Could you check a few things on this model? Use its own coordinates, in mm. Give positions to 0.01 mm unless a question says otherwise; leave off trailing zeros. Order: outer loops, then holes, each group sorted by start corner. A loop starts at its lowest first (then second) coordinate and runs counter-clockwise, first axis right, second up. Notation, with made-up numbers: M 48.25,31.25 L 107.25,31.25 A22 ccw 107.25,43.25 Z; hole C 49,85.5 d5. An arc over 180 degrees is marked long. Use a Markdown table: item, result. Add a question column.
Autodesk Inventor part; units mm, degrees
ref_plane "NUT_XY" through (0, 0, 0) normal (0, 0, 1) x (1, 0, 0)
ref_plane "NUT_YZ" through (0, 0, 0) normal (1, 0, 0) x (0, 1, 0)
ref_plane "NUT_ZX" through (0, 0, 0) normal (0, 1, 0) x (0, 0, 1)
sketch "Sketch_8" plane through (0, 0, 0) normal (1, 0, 0) x (0, 1, 0)
  line L0 (0, -4.064) -> (0, 0)
  line L1 (0, 0) -> (5.588, 0)
  line L2 (5.588, 0) -> (6.7056, -0.2995)
  line L3 (6.7056, -0.2995) -> (6.7056, -3.7645)
  line L4 (6.7056, -3.7645) -> (5.588, -4.064)
  line L5 (5.588, -4.064) -> (0, -4.064)
  line L6 (0, -4.064) -> (0, 0)
sketch "Sketch_10" plane through (0, 0, 0) normal (0, 0, 1) x (1, 0, 0)
  line L0 (-11.176, 11.176) -> (-11.176, -11.176)
  line L1 (-11.176, -11.176) -> (11.176, -11.176)
  line L2 (11.176, -11.176) -> (11.176, 11.176)
  line L3 (11.176, 11.176) -> (-11.176, 11.176)
  line L4 (-5.588, 3.2262) -> (-5.588, -3.2262)
  line L5 (-5.588, -3.2262) -> (0, -6.4525)
  line L6 (0, -6.4525) -> (5.588, -3.2262)
  line L7 (5.588, -3.2262) -> (5.588, 3.2262)
  line L8 (5.588, 3.2262) -> (0, 6.4525)
  line L9 (0, 6.4525) -> (-5.588, 3.2262)
revolve "Revolution1" add sketch "Sketch_8" angle 360 about axis through (0, 0, -4.064) along (0, 0, -1)
extrude "Extrusion1" cut sketch "Sketch_10" against normal blind 4.064
sketch "Sketch_11" plane through (0, 0, 0) normal (1, 0, 0) x (0, 1, 0)
  line L0 (0, -4.064) -> (0, 0)
  line L1 (0, 0) -> (3.175, 0)
  line L2 (3.175, 0) -> (2.6835, -0.4915)
  line L3 (2.6835, -0.4915) -> (2.6835, -3.5725)
  line L4 (2.6835, -3.5725) -> (3.175, -4.064)
  line L5 (3.175, -4.064) -> (0, -4.064)
  line L6 (0, -4.064) -> (0, 0)
revolve "Revolution2" cut sketch "Sketch_11" angle 360 about axis through (0, 0, -4.064) along (0, 0, -1)
thread "Thread1"
ref_plane "NUT_XY" through (0, 0, 0) normal (0, 0, 1) x (1, 0, 0)
ref_plane "NUT_YZ" through (0, 0, 0) normal (1, 0, 0) x (0, 1, 0)
ref_plane "NUT_ZX" through (0, 0, 0) normal (0, 1, 0) x (0, 0, 1)
ref_plane "a1_XY" through (-5.588, 5.588, 0) normal (0, 0, 1) x (1, 0, 0)
ref_plane "a1_YZ" through (-5.588, 5.588, 0) normal (1, 0, 0) x (0, 1, 0)
ref_plane "a1_ZX" through (-5.588, 5.588, 0) normal (0, 1, 0) x (0, 0, 1)
ref_plane "a2_XY" through (5.588, 5.588, 0) normal (0, 0, 1) x (1, 0, 0)
ref_plane "a2_YZ" through (5.588, 5.588, 0) normal (1, 0, 0) x (0, 1, 0)
ref_plane "a2_ZX" through (5.588, 5.588, 0) normal (0, 1, 0) x (0, 0, 1)
ref_plane "b1_XY" through (0, 5.588, 0) normal (1, 0, 0) x (0, 0, -1)
ref_plane "b1_YZ" through (0, 5.588, 0) normal (0, 0, -1) x (0, 1, 0)
ref_plane "b1_ZX" through (0, 5.588, 0) normal (0, 1, 0) x (1, 0, 0)
ref_plane "b2_XY" through (0, 5.588, -4.064) normal (1, 0, 0) x (0, 0, -1)
ref_plane "b2_YZ" through (0, 5.588, -4.064) normal (0, 0, -1) x (0, 1, 0)
ref_plane "b2_ZX" through (0, 5.588, -4.064) normal (0, 1, 0) x (1, 0, 0)
ref_plane "e_XY" through (0, 0, -4.064) normal (1, 0, 0) x (0, 0, -1)
ref_plane "e_YZ" through (0, 0, -4.064) normal (0, 0, -1) x (0, 1, 0)
ref_plane "e_ZX" through (0, 0, -4.064) normal (0, 1, 0) x (1, 0, 0)
ref_plane "th1_XY" through (0, 3.175, -4.064) normal (1, 0, 0) x (0, 0, -1)
ref_plane "th1_YZ" through (0, 3.175, -4.064) normal (0, 0, -1) x (0, 1, 0)
ref_plane "th1_ZX" through (0, 3.175, -4.064) normal (0, 1, 0) x (1, 0, 0)
ref_plane "th2_XY" through (0, -3.175, -4.064) normal (1, 0, 0) x (0, 0, -1)
ref_plane "th2_YZ" through (0, -3.175, -4.064) normal (0, 0, -1) x (0, 1, 0)
ref_plane "th2_ZX" through (0, -3.175, -4.064) normal (0, 1, 0) x (1, 0, 0)
ref_plane "ol1_XY" through (0, 0, -5.588) normal (0, 1, 0) x (1, 0, 0)
ref_plane "ol1_YZ" through (0, 0, -5.588) normal (1, 0, 0) x (0, 0, -1)
ref_plane "ol1_ZX" through (0, 0, -5.588) normal (0, 0, -1) x (0, 1, 0)
ref_plane "ol2_XY" through (4.064, 0, -5.588) normal (0, 1, 0) x (1, 0, 0)
ref_plane "ol2_YZ" through (4.064, 0, -5.588) normal (1, 0, 0) x (0, 0, -1)
ref_plane "ol2_ZX" through (4.064, 0, -5.588) normal (0, 0, -1) x (0, 1, 0)
properties part number "D-344"
1) Please list where these lines run through material, in increasing order: line 1 (X direction, y = 0, z = -2.25); line 2 (X direction, y = 0.5, z = -0.95); line 3 (Y direction, x = 1.75, z = -1.1). Write a range as from..to.
2) Suppose I cut it at A-A on z = -2.2. Please give me the cut outline in (x, y).
3) For pin 1 (1 mm diameter, centred on x = 4, z = -2.5, fed in from -Y), with a flat end and sliding along its axis, tell me the tip position at first contact or that it passes through.
Values found:
| question | item | result |
|---|---|---|
| 1 | line 1 | x = -5.59..-2.68, 2.68..5.59 |
| 1 | line 2 | x = -5.59..-2.64, 2.64..5.59 |
| 1 | line 3 | y = -5.44..-2.03, 2.03..5.44 |
| 2 | outline | M -5.59,-3.23 L 0,-6.45 L 5.59,-3.23 L 5.59,3.23 L 0,6.45 L -5.59,3.23 Z; hole C 0,0 d5.37 |
| 3 | pin 1 | stops at y = -4.43 |
